For this review, take the finished solid that the model builds, in its own axes (mm). A direction names the side the tool comes from. Give positions to 0.01 mm unless a question says otherwise; leave off trailing zeros. Write each loop counter-clockwise with the first axis right and the second up, starting at its lowest first coordinate (ties: lowest second). Pieces come first, ordered by that corner, then holes. Notation, with made-up numbers: M 8,67 L 62,67 A14 ccw 62,91 Z; hole C 1,51 d10. An arc over 180 degrees is marked long. Use one line per item in the form item = value. Start each with the question number.
Q1. Consider section A-A on z = -5.5. Write out the cut boundary in (x, y), and give its area (3 significant figures).
Q2. Consider section B-B on x = 164. Write out the cut boundary in (y, z) (3 decimals), and give its area (3 significant figures).
Q3. Consider section C-C on y = 6.5. Write out the cut boundary in (x, z) (3 decimals), and give its area (3 significant figures).
Q4. Clearance check with flat-ended pins moving along their axes: pin 1 Ø10 at (y, z) = (13, 8) entering from +X; pin 2 Ø10 at (y, z) = (-18, 9) entering from -X. State where each tip first meets the part, or that it passes through.
Q5. Tool access review of faces 1 (the flat face through (-4, -23.614, 0)), 2 (the flat face through (381, 0, 13)): name each direction out of +Z, -Z, +X, -X, +Y, -Y from which nothing blocks a thin tool from reaching the whole face with its end or side.
Q6. For probe 1 along Y at (x, z) = (93, 11); probe 2 along Y at (x, z) = (-285, 9.25); probe 3 along Z at (x, y) = (53, -8), list the stretches that pass through material, from the lowest coordinate up. Write a range as [from, to].
Q7. Consider section D-D on x = 359.5. Write out the cut boundary in (y, z) (3 decimals), and give its area (3 significant figures).
```python
from build123d import *

# Parameters (mm, degrees)
BOSS_EXTRUDE1_DEPTH      = 13.49375
BOSS_EXTRUDE1_DEPTH_BACK = 13.49375
CUT_EXTRUDE1_DEPTH       = 414.750895817
CUT_EXTRUDE1_DEPTH_BACK  = 414.750895817
SKETCH3_W                = 23.6140625
SKETCH3_H                = 47.228125
FILLET1_R                = 1.27
FILLET2_R                = 0.635


with BuildPart() as part:
    # Sketch2 → Boss-Extrude1 (new, two sides: drawn at the far end of the back side and taken through both)
    with BuildSketch(Plane.XY.offset(-BOSS_EXTRUDE1_DEPTH_BACK)):
        Polygon((-349.25, -25.4), (-387.383370876, 25.4), (-349.25, 25.4), (349.25, 25.4), (412.75, 25.4), (349.25, -25.4), align=None)
    extrude(amount=BOSS_EXTRUDE1_DEPTH + BOSS_EXTRUDE1_DEPTH_BACK)

    # Sketch3 → Cut-Extrude1 (cut, two sides: drawn at the far end of the back side and taken through both)
    with BuildSketch(Plane(origin=(0, 0, 0), x_dir=(0, 0, -1), z_dir=(1, 0, 0)).offset(-CUT_EXTRUDE1_DEPTH_BACK)):
        Rectangle(SKETCH3_W, SKETCH3_H)
    extrude(amount=CUT_EXTRUDE1_DEPTH + CUT_EXTRUDE1_DEPTH_BACK, mode=Mode.SUBTRACT)

    # Fillet1
    fillet1_edges = [part.edges().sort_by_distance(p)[0] for p in [
        (0.445897778, -23.6140625, -11.80703125),
        (0.445897778, -23.6140625, 11.80703125),
        (12.237416785, 23.6140625, 11.80703125),
        (12.237416785, 23.6140625, -11.80703125),
    ]]
    fillet(fillet1_edges, radius=FILLET1_R)

    # Fillet2
    fillet2_edges = [part.edges().sort_by_distance(p)[0] for p in [
        (12.683314562, 25.4, 13.49375),
        (0, -25.4, 13.49375),
        (0, -25.4, -13.49375),
        (12.683314562, 25.4, -13.49375),
    ]]
    fillet(fillet2_edges, radius=FILLET2_R)


solid = part.part
```
Working result:
q1.outline = M -387.38,25.4 L -386.04,23.61 L 410.52,23.61 L 412.75,25.4 Z; M -350.59,-23.61 L -349.25,-25.4 L 349.25,-25.4 L 351.48,-23.61 Z
q1.area = 2,680 mm²
q2.outline = M -25.4,-12.859 A0.635 ccw -24.765,-13.494 L 24.765,-13.494 A0.635 ccw 25.4,-12.859 L 25.4,12.859 A0.635 ccw 24.765,13.494 L -24.765,13.494 A0.635 ccw -25.4,12.859 Z; hole M -23.614,-10.537 A1.27 ccw -22.344,-11.807 L 22.344,-11.807 A1.27 ccw 23.614,-10.537 L 23.614,10.537 A1.27 ccw 22.344,11.807 L -22.344,11.807 A1.27 ccw -23.614,10.537 Z
q2.area = 257 mm²
q3.outline = M -373.196,-13.494 L 389.125,-13.494 L 389.125,-11.807 L -373.196,-11.807 Z; M -373.196,11.807 L 389.125,11.807 L 389.125,13.494 L -373.196,13.494 Z
q3.area = 2,570 mm²
q4.pin_1 = 401.3
q4.pin_2 = -357.91
q5.face_1 = +X, -X
q5.face_2 = +Z, -Z, +X, -Y
q6.probe_1 = [-25.4, -23.53], [23.53, 25.4]
q6.probe_2 = [-25.4, -23.61], [23.61, 25.4]
q6.probe_3 = [-13.49, -11.81], [11.81, 13.49]
q7.outline = M -17.2,-13.494 L 24.765,-13.494 A0.635 ccw 25.4,-12.859 L 25.4,12.859 A0.635 ccw 24.765,13.494 L -17.2,13.494 L -17.2,11.807 L 22.344,11.807 A1.27 cw 23.614,10.537 L 23.614,-10.537 A1.27 cw 22.344,-11.807 L -17.2,-11.807 Z
q7.area = 186 mm²
